from build123d import *

# Parameters (mm, degrees)
SKETCH1_W                     = 25
SKETCH1_H                     = 15
BOSS_EXTRUDE1_DEPTH           = 5.026
M2_TAPPED_HOLE1_D             = 1.6
M2_TAPPED_HOLE1_DEPTH         = 3.5
M2_TAPPED_HOLE1_TIP           = 0.480688495
SKETCH5_R                     = 15
BOSS_EXTRUDE2_DEPTH           = 7.5
SKETCH6_R                     = 12.25
CUT_EXTRUDE1_DEPTH            = 5.25
F_1_1_8_12_TAPPED_HOLE2_D     = 25.4
F_1_1_8_12_TAPPED_HOLE2_DEPTH = 6.25
CUT_EXTRUDE2_DEPTH            = 3.5
SKETCH14_W                    = 8
SKETCH14_H                    = 1.5
CUT_EXTRUDE3_DEPTH            = 13.5
SKETCH15_R                    = 6
CUT_EXTRUDE4_DEPTH            = 13.5


with BuildPart() as part:
    # Sketch1 → Boss-Extrude1 (new body)
    with BuildSketch(Plane.XY):
        with Locations((12.5, 7.5)):
            Rectangle(SKETCH1_W, SKETCH1_H)
    extrude(amount=BOSS_EXTRUDE1_DEPTH)

    # M2 Tapped Hole1
    with Locations(Plane(origin=(0, 0, 0), x_dir=(-1, 0, 0), z_dir=(0, 0, -1))):
        with Locations((-23, 7.5), (-2, 7.5)):
            Hole(M2_TAPPED_HOLE1_D / 2, depth=M2_TAPPED_HOLE1_DEPTH)
            with Locations((0, 0, -(M2_TAPPED_HOLE1_DEPTH + M2_TAPPED_HOLE1_TIP / 2))):  # 118° drill point
                Cone(0, M2_TAPPED_HOLE1_D / 2, M2_TAPPED_HOLE1_TIP, mode=Mode.SUBTRACT)

    # Sketch5 → Boss-Extrude2 (add)
    with BuildSketch(Plane.XY.offset(5.026)):
        with Locations((12.5, 7.75)):
            Circle(SKETCH5_R)
    extrude(amount=BOSS_EXTRUDE2_DEPTH)

    # Sketch6 → Cut-Extrude1 (cut)
    with BuildSketch(Plane.XY.offset(12.526)):
        with Locations((12.5, 7.75)):
            Circle(SKETCH6_R)
    extrude(amount=-CUT_EXTRUDE1_DEPTH, mode=Mode.SUBTRACT)

    # 1-1/8-12 Tapped Hole2
    with Locations(Plane.XY.offset(12.526)):
        with Locations((12.5, 7.75)):
            Hole(F_1_1_8_12_TAPPED_HOLE2_D / 2, depth=F_1_1_8_12_TAPPED_HOLE2_DEPTH)

    # Sketch13 → Cut-Extrude2 (cut)
    with BuildSketch(Plane(origin=(0, 0, 0), x_dir=(-1, 0, 0), z_dir=(0, 0, -1))):
        Polygon((-12.5, 3.75), (-12.5, 7.5), (-12.5, 7.75), (-12.5, 11.75), (-16.5, 11.75), (-16.5, 3.75), align=None)
        Polygon((-12.5, 7.75), (-12.5, 7.5), (-12.5, 3.75), (-8.5, 3.75), (-8.5, 11.75), (-12.5, 11.75), align=None)
    extrude(amount=-CUT_EXTRUDE2_DEPTH, mode=Mode.SUBTRACT)

    # Sketch14 → Cut-Extrude3 (cut)
    with BuildSketch(Plane(origin=(0, 3.75, 0), x_dir=(1, 0, 0), z_dir=(0, 1, 0))):
        with Locations((12.5, -0.75)):
            Rectangle(SKETCH14_W, SKETCH14_H)
    extrude(amount=-CUT_EXTRUDE3_DEPTH, mode=Mode.SUBTRACT)

    # Sketch15 → Cut-Extrude4 (cut)
    with BuildSketch(Plane(origin=(0, 0, 3.5), x_dir=(-1, 0, 0), z_dir=(0, 0, -1))):
        with Locations((-12.5, 7.75)):
            Circle(SKETCH15_R)
    extrude(amount=-CUT_EXTRUDE4_DEPTH, mode=Mode.SUBTRACT)


solid = part.part
Check sheet for the modelled part. Datum: model origin and axes. Units: mm. A direction names the side the tool comes from. Round coordinates to 2 decimals unless told otherwise and drop trailing zeros. Loops run counter-clockwise (first coordinate to the right, second up) from the corner with the lowest first, then second, coordinate; pieces in that order, holes last. Notation, with made-up numbers: (49, 74.5) -> (87, 74.5) arc R11 ccw to (87, 94.5) -> close; hole circle Ø6 at (-31.75, 73.25). An arc over 180 degrees is marked (long way). Put each result on its own line as item: value. Start each with the question number.
1. Draft check along Y on faces 1 (the face through (22.578, 0.022, 9.357)), 2 (the face through (12, 0, 2)), 3 (the face through (25, 7, 2)). Enter one of: +Y half, -Y half, draft (parallel to the pull), parting line (faces both ways), or undercut.
2. Section check B-B (z = 3). Enter the section's corners in (x, y).
3. Scan lines: probe 1 along X at (y, z) = (7.5, 2.45); probe 2 along Y at (x, z) = (11.25, 3); probe 3 along Y at (x, z) = (23, 2.2). Record each from-to range of solid material in increasing order.
4. Section check C-C (y = 6). Enter the section's corners in (x, z), plus the area to 3 significant figures.
5. Access from +Z, -Z, +X, -X, +Y, -Y to the whole of each face (thin tool, end or side, straight path). Record for faces 4 (the face through (0, 7, 2)), 5 (the face through (17, 7, 3.5)), 6 (the face through (12, 15, 2)), 7 (the face through (8.5, 7, 2)), 8 (the face through (13, 3.75, 2)).
6. Section check A-A (x = 12.5). Enter the section's corners in (y, z).
7. Gauge pin test, flat ends, axial feed: pin 1 (2 mm diameter, centred on x = 2, y = 7.5, fed in from +Z); pin 2 (4 mm diameter, centred on y = 7, z = 2, fed in from +X); pin 3 (6 mm diameter, centred on y = 18.5, z = 6, fed in from +X). Record the tip position at first contact, or that the pin passes through.
8. Section check D-D (y = -2). Enter the section's corners in (x, z).
Findings:
1. face 1: undercut
1. face 2: -Y half
1. face 3: draft
2. outline: (0, 0) -> (25, 0) -> (25, 15) -> (0, 15) -> close; hole circle Ø1.6 at (2, 7.5); hole (8.5, 3.75) -> (16.5, 3.75) -> (16.5, 11.75) -> (8.5, 11.75) -> close; hole circle Ø1.6 at (23, 7.5)
3. probe 1: x = 0 to 1.2, 2.8 to 8.5, 16.5 to 22.2, 23.8 to 25
3. probe 2: y = 0 to 3.75, 11.75 to 15
3. probe 3: y = 0 to 6.7, 8.3 to 15
4. outline: (-2.4, 5.03) -> (0, 5.03) -> (0, 0) -> (8.5, 0) -> (8.5, 3.5) -> (6.76, 3.5) -> (6.76, 6.28) -> (-0.08, 6.28) -> (-0.08, 12.53) -> (-2.4, 12.53) -> close; (16.5, 0) -> (25, 0) -> (25, 5.03) -> (27.4, 5.03) -> (27.4, 12.53) -> (25.08, 12.53) -> (25.08, 6.28) -> (18.24, 6.28) -> (18.24, 3.5) -> (16.5, 3.5) -> close
4. area: 132 mm^2
5. face 4: -Z, -X, +Y, -Y
5. face 5: +Z
5. face 6: -Z, +X, -X, +Y
5. face 7: -Z
5. face 8: +Z, -Z
6. outline: (-7.25, 5.03) -> (0, 5.03) -> (0, 1.5) -> (3.75, 1.5) -> (3.75, 3.5) -> (1.75, 3.5) -> (1.75, 6.28) -> (-4.95, 6.28) -> (-4.95, 12.53) -> (-7.25, 12.53) -> close; (11.75, 0) -> (15, 0) -> (15, 5.03) -> (22.75, 5.03) -> (22.75, 12.53) -> (20.45, 12.53) -> (20.45, 6.28) -> (13.75, 6.28) -> (13.75, 3.5) -> (11.75, 3.5) -> close
7. pin 1: stops at z = 6.28
7. pin 2: stops at x = 25
7. pin 3: stops at x = 25.34
8. outline: (1.1, 5.03) -> (23.9, 5.03) -> (23.9, 12.53) -> (20.64, 12.53) -> (20.64, 6.28) -> (4.36, 6.28) -> (4.36, 12.53) -> (1.1, 12.53) -> close
